Can you work these out from the drawing? Everything is in mm from the part's minimum corner. Round coordinates to 2 decimals unless told otherwise and drop trailing zeros. Loops run counter-clockwise (first coordinate to the right, second up) from the corner with the lowest first, then second, coordinate; pieces in that order, holes last. Notation, with made-up numbers: M 12,84.25 L 59,84.25 A16 cw 59,106.25 Z; hole C -34.5,84.5 d11. An arc over 180 degrees is marked long. One line per question, with ' | ' between items. Start each with the question number.
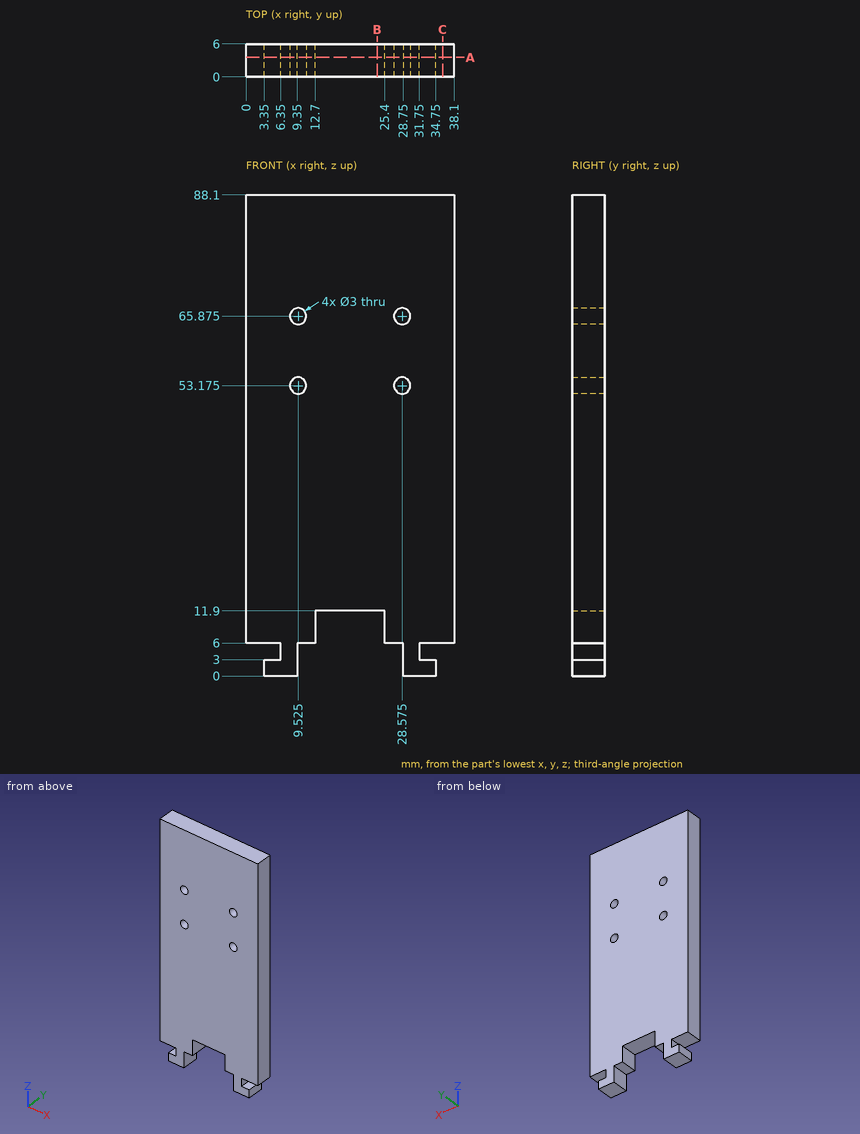
1) Please list where these lines run through material, in increasing order: L1, parallel to X at y = 1.25, z = 54; L2, parallel to Z at x = 5.5, y = 3.7; L3, parallel to Z at x = 29, y = 0.3. Write a range as from..to.
2) I'm going to push flat-ended pins straight in: pin 1 Ø0.9 at (y, z) = (4.5, 4) entering from -X; pin 2 Ø0.9 at (y, z) = (2.5, 4.5) entering from +X; pin 3 Ø3.5 at (y, z) = (3, 1.5) entering from -X. Where does each tip first touch, or does it pass through?
3) Imagine slicing it at A-A (y = 3.55). Write out the boundary of the cut face in (x, z) (3 decimals).
4) Imagine slicing it at B-B (x = 24). Write out the boundary of the cut face in (y, z).
5) Imagine slicing it at C-C (x = 36). Write out the boundary of the cut face in (y, z).
Results are:
1) L1: 0..8.27, 10.78..27.32, 29.83..38.1 | L2: 0..3, 6..88.1 | L3: 0..51.74, 54.61..64.44, 67.31..88.1
2) pin 1: x = 6.35 | pin 2: x = 31.75 | pin 3: x = 3.35
3) outline: M 0,6 L 6.35,6 L 6.35,3 L 3.35,3 L 3.35,0 L 9.35,0 L 9.35,6 L 12.7,6 L 12.7,11.9 L 25.4,11.9 L 25.4,6 L 28.75,6 L 28.75,0 L 34.75,0 L 34.75,3 L 31.75,3 L 31.75,6 L 38.1,6 L 38.1,88.1 L 0,88.1 Z; hole C 9.525,53.175 d3; hole C 9.525,65.875 d3; hole C 28.575,53.175 d3; hole C 28.575,65.875 d3
4) outline: M 0,11.9 L 6,11.9 L 6,88.1 L 0,88.1 Z
5) outline: M 0,6 L 6,6 L 6,88.1 L 0,88.1 Z
